Source: CAD feature listing. Evaluate the final solid. Frame: model axes, mm. A direction names the side the tool comes from. Give positions to 0.01 mm unless a question says otherwise; leave off trailing zeros. Write each loop counter-clockwise with the first axis right and the second up, starting at its lowest first coordinate (ties: lowest second). Pieces come first, ordered by that corner, then holes. Notation, with made-up numbers: (-32, -13.5) -> (-15, -13.5) arc R19 ccw to (-15, 12.5) -> close; hole circle Ø6 at (28, 42.25). An arc over 180 degrees is marked (long way). Use one line per item in the form item = value. Start each with the question number.
(1) Draft query along X for faces 5 (the face through (9, -5, -74.65)), 6 (the face through (-10.58, -0.33, -50.38)), 7 (the face through (8.87, 4.49, -6.62)). Return one class per face: pulls with the +X half, pulls with the -X half, needs draft (parallel to the pull), parting line crosses it, or undercut.
(2) Material intervals for line 1 along Y through (x, z) = (9, -74.5) (3 decimals); line 2 along Z through (x, y) = (6, 0); line 3 along Y through (x, z) = (9, -75.25) (3 decimals), sorted ascending. Write a range as from..to.
(3) Cut plane D-D, the plane z = -26.5. Output: boundary loops of the cut face in (x, y).
(4) Cut plane B-B, the plane z = -65. Output: boundary loops of the cut face in (x, y), and give its area (3 significant figures).
(5) Cut plane C-C, the plane z = 13. Output: boundary loops of the cut face in (x, y), and give its area (3 significant figures).
(6) First-contact query: P1, Ø6, axis at x = 7.5, y = 4, coming from the +Z side; P2, Ø24, axis at y = -2, z = -55, coming from the -X side; P3, Ø21.5, axis at y = -7, z = -8, coming from the -X side; P4, Ø8, axis at y = 0, z = 0, coming from the -X side. Flat tips, straight axial feed; report the tip coordinate or a pass-through.
(7) Cut plane A-A, the plane x = 1.5. Output: boundary loops of the cut face in (y, z), and give its area (3 significant figures).
(8) Set-up query: faces 1 (the face through (9, 0, -38)), 2 (the face through (9, 12.5, -76.5)), 3 (the face through (0, 0, 7)), 4 (the face through (28.716, -0.326, -50.905)). Return all of +Z, -Z, +X, -X, +Y, -Y with unobstructed straight access to the full face (end or side cutting, diameter ignored); none if empty.
Autodesk Inventor part; units mm, degrees
ref_plane "YZ Plane" through (0, 0, 0) normal (1, 0, 0) x (0, 1, 0)
ref_plane "XZ Plane" through (0, 0, 0) normal (0, 1, 0) x (-1, 0, 0)
ref_plane "XY Plane" through (0, 0, 0) normal (0, 0, 1) x (1, 0, 0)
sketch "Sketch28" plane through (0, 0, 0) normal (1, 0, 0) x (0, 1, 0)
  circle A0 centre (0, 0) radius 6.5
  arc A1 (23.289, 0) -> (-23.289, 0) centre (0, 0) ccw
  line L0 (23.289, 0) -> (23.289, -80)
  line L1 (-23.289, 0) -> (-23.289, -80)
  line L2 (23.289, -80) -> (-23.289, -80)
  dimension "d103" = 13
  dimension "d104" = 46.578
  dimension "d105" = 80
  dimension "d106" = 80
extrude "Extrusion23" add sketch "Sketch28" along normal blind 18
sketch "Sketch29" plane through (0, 23.289, 0) normal (0, 1, 0) x (1, 0, 0)
  line L0 (31.5, 80) -> (-13.5, 80)
  line L1 (-13.5, 80) -> (-13.5, 45)
  line L2 (-13.5, 45) -> (31.5, 45)
  line L3 (31.5, 45) -> (31.5, 80)
  line L4 (0, 80) -> (18, 80)
  line L5 (18, 0) -> (18, 80)
  arc A0 (31.5, 45) -> (18, 20) centre (57.6517, 14.7331) ccw
  line L6 (9, 88.5963) -> (9, -26.2001) construction
  arc A1 (0, 20) -> (-13.5, 45) centre (-39.6517, 14.7331) ccw
  line L7 (0, 80) -> (0, 0)
  point P0 (9, 80)
  point P1 (9, 45)
  point P2 (0, 45)
  point P3 (18, 45)
  dimension "d109" = 45
  dimension "d110" = 0
  dimension "d111" = 35
  dimension "d112" = 22.5
  dimension "d115" = 40
  dimension "d116" = 25
extrude "Extrusion24" add sketch "Sketch29" against normal up to surface (46.578 mm away)
fillet "Fillet9" radius 90 2 edges at (31.5, 0, -45) (-13.5, 0, -45)
sketch "Sketch30" plane through (0, 23.289, 0) normal (0, 1, 0) x (1, 0, 0)
  line L0 (19, 73) -> (-1, 73)
  line L1 (-1, 73) -> (-1, 38)
  line L2 (-1, 38) -> (19, 38)
  line L3 (19, 38) -> (19, 73)
  line L4 (-13.5, 80) -> (31.5, 80)
  point P0 (0, 0)
  dimension "d120" = 7
  dimension "d121" = 20
  dimension "d122" = 12.5
  dimension "d123" = 35
extrude "Extrusion25" cut sketch "Sketch30" against normal through all
fillet "Fillet10" radius 5 2 edges at (19, 0, -38) (-1, 0, -38)
fillet "Fillet11" radius 10 2 edges at (-13.5, 0, -80) (31.5, 0, -80)
sketch "Sketch31" plane through (21.4392, -23.289, -80) normal (0, 0, -1) x (-1, 0, 0)
  arc A0 (15.3892, 23.5545) -> (9.4892, 23.5545) centre (12.4392, 28.664) ccw
  line L0 (15.3892, 23.5545) -> (15.3892, 22.764)
  arc A1 (9.4892, 22.764) -> (15.3892, 22.764) centre (12.4392, 22.764) ccw
  line L1 (9.4892, 22.764) -> (9.4892, 23.5545)
  point P0 (21.4392, 23.289)
extrude "Extrusion26" cut sketch "Sketch31" against normal blind 20
sketch "Sketch34" plane through (-1, 23.289, -73) normal (0, 0, 1) x (1, 0, 0)
  line L0 (3.925, -12.014) -> (16.075, -12.014)
  line L1 (16.075, -12.014) -> (16.075, -34.564)
  line L2 (16.075, -34.564) -> (3.925, -34.564)
  line L3 (3.925, -34.564) -> (3.925, -12.014)
  line L4 (1, 0) -> (19, 0)
  arc A0 (12.95, -23.0235) -> (7.05, -23.0235) centre (10, -17.914) ccw
  point P0 (1, -23.289)
  point P1 (10, 0)
  dimension "d130" = 12.014
  dimension "d131" = 22.55
  dimension "d132" = 12.15
  dimension "d133" = 6.075
extrude "Extrusion27" cut sketch "Sketch34" against normal blind 1.65
sketch "Sketch36" plane through (-1, 23.289, -73) normal (0, 0, 1) x (1, 0, 0)
  arc A0 (10.5833, -38.1445) -> (9.4167, -38.1445) centre (10, -37.039) ccw
  arc A1 (9.4167, -8.4335) -> (10.5833, -8.4335) centre (10, -9.539) ccw
  circle A2 centre (10, -9.539) radius 1.25
  circle A3 centre (10, -37.039) radius 1.25
  point P0 (1, -23.289)
  point P1 (10.5833, -8.4335)
  point P2 (9.4167, -8.4335)
  point P3 (9.4167, -38.1445)
  point P4 (10.5833, -38.1445)
extrude "Extrusion28" cut sketch "Sketch36" against normal through all
sketch "Sketch37" plane through (0, 0, 0) normal (-1, 0, 0) x (0, 0, 1)
  line L0 (-6.3739, 1.2741) -> (-8.0335, 2.3902)
  line L1 (-3.5835, 5.423) -> (-5.243, 6.5392)
  line L2 (-5.243, 6.5392) -> (-8.0335, 2.3902)
  circle A0 centre (0, 0) radius 6.5
extrude "Extrusion29" cut sketch "Sketch37" against normal through all
sketch "Sketch38" plane through (0, 23.289, 0) normal (0, 1, 0) x (1, 0, 0)
  line L0 (-25.331, 0) -> (24.4324, 0)
  line L1 (0, 0) -> (18, 0)
  line L2 (9, 31.2847) -> (9, -25.5557)
  line L3 (0, -23.289) -> (18, -23.289)
  line L4 (14, 38) -> (4, 38)
  arc A0 (-1, 43) -> (4, 38) centre (4, 43) ccw
  line L5 (-1, 43) -> (-1, 73)
  line L6 (-1, 73) -> (19, 73)
  line L7 (19, 73) -> (19, 43)
  arc A1 (14, 38) -> (19, 43) centre (14, 43) ccw
  arc A2 (31.4316, 69.6103) -> (21.4392, 80) centre (21.4392, 70) ccw
  line L8 (-3.4392, 80) -> (21.4392, 80)
  arc A3 (-3.4392, 80) -> (-13.4316, 69.6103) centre (-3.4392, 70) ccw
  arc A4 (-13.4316, 69.6103) -> (-3.9127, 32.6976) centre (76.5, 73.1178) ccw
  arc A5 (0, 20) -> (-3.9127, 32.6976) centre (-39.6517, 14.7331) ccw
  line L9 (0, 20) -> (0, 0)
  line L10 (0, 0) -> (18, 0)
  line L11 (18, 20) -> (18, 0)
  arc A6 (21.9127, 32.6976) -> (18, 20) centre (57.6517, 14.7331) ccw
  arc A7 (21.9127, 32.6976) -> (31.4316, 69.6103) centre (-58.5, 73.1178) ccw
  circle A8 centre (9, 0) radius 2.5
  dimension "d140" = 0
  dimension "d141" = 9
  dimension "d142" = 5
properties part number "Link Three" material "ABS Plastic"
Geometry says:
q1.face_5 = undercut
q1.face_6 = pulls with the -X half
q1.face_7 = needs draft
q2.line_1 = -23.289..-15, -12.5..-11.275, 11.275..12.5, 15..23.289
q2.line_2 = -80..-74.65, -38..-6.5, 6.5..23.29
q2.line_3 = -23.289..-15, -12.5..-3.475, 11.275..12.5, 15..23.289
q3.outline = (-1.42, -23.29) -> (19.42, -23.29) -> (19.42, 23.29) -> (-1.42, 23.29) -> close
q4.outline = (-13.13, -23.29) -> (-1, -23.29) -> (-1, 23.29) -> (-13.13, 23.29) -> close; (19, -23.29) -> (31.13, -23.29) -> (31.13, 23.29) -> (19, 23.29) -> close
q4.area = 1,130 mm^2
q5.outline = (0, -19.32) -> (18, -19.32) -> (18, 19.32) -> (0, 19.32) -> close
q5.area = 696 mm^2
q6.P1 = 23.27
q6.P2 = -13.29
q6.P3 = 0
q6.P4 = through
q7.outline = (-23.29, -80) -> (23.29, -80) -> (23.29, -73) -> (-23.29, -73) -> close; (-23.29, -38.67) -> (23.29, -38.67) -> (23.29, 0) arc R23.29 ccw to (-23.29, 0) -> close; hole (1.27, -6.37) -> (2.39, -8.03) -> (6.54, -5.24) -> (5.42, -3.58) arc R6.5 ccw (long way) to start
q7.area = 2,840 mm^2
q8.face_1 = +Y, -Y
q8.face_2 = -Z
q8.face_3 = +Z, -X, +Y, -Y
q8.face_4 = +Z, +X, +Y, -Y
